Geometry: final body of the model. Coordinates: model frame, mm. Face numbers are marked on the shaded views. Give positions to 0.01 mm unless a question says otherwise; leave off trailing zeros. Loops run counter-clockwise (first coordinate to the right, second up) from the corner with the lowest first, then second, coordinate; pieces in that order, holes last. Notation, with made-up numbers: M 6,56 L 11,56 A22 cw 11,67 Z; hole C 56.5,-11.75 d8. An arc over 180 degrees is marked long. Put each result on its own line as item: value.
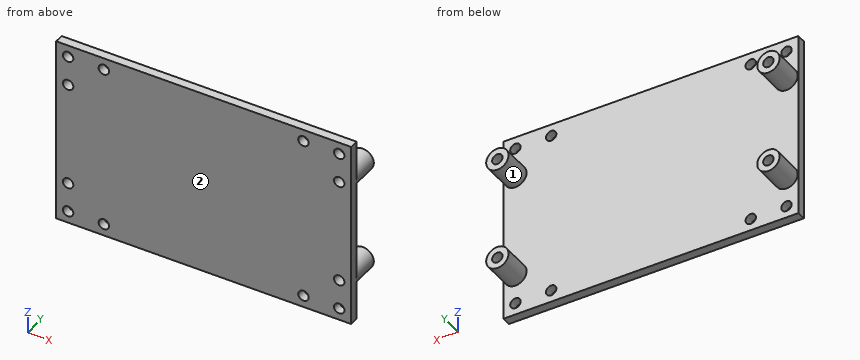
```python
from build123d import *

# Parameters (mm, degrees)
SKETCH1_W           = 99
SKETCH1_H           = 63
SKETCH1_R           = 3.75
SKETCH1_R_2         = 1.75
BOSS_EXTRUDE1_DEPTH = 3
SKETCH1_3_R         = 3.75
SKETCH1_3_R_2       = 1.75
BOSS_EXTRUDE2_DEPTH = 13


with BuildPart() as part:
    # Sketch1 → Boss-Extrude1 (new body)
    with BuildSketch(Plane(origin=(0, 0, 0), x_dir=(1, 0, 0), z_dir=(0, 1, 0))):
        Rectangle(SKETCH1_W, SKETCH1_H)
        with Locations(Location((-45.5, -17.5, 0), (0, 0, 270))):
            Circle(SKETCH1_R, mode=Mode.SUBTRACT)
        with Locations(Location((45.5, -17.5, 0), (0, 0, 270))):
            Circle(SKETCH1_R, mode=Mode.SUBTRACT)
        with Locations(Location((-45.5, 17.5, 0), (0, 0, 270))):
            Circle(SKETCH1_R, mode=Mode.SUBTRACT)
        with Locations(Location((45.5, 17.5, 0), (0, 0, 270))):
            Circle(SKETCH1_R, mode=Mode.SUBTRACT)
        with Locations(Location((45.5, 27.5, 0), (0, 0, 270))):
            Circle(SKETCH1_R_2, mode=Mode.SUBTRACT)
        with Locations(Location((-45.5, 27.5, 0), (0, 0, 270))):
            Circle(SKETCH1_R_2, mode=Mode.SUBTRACT)
        with Locations(Location((-33.5, 27.5, 0), (0, 0, 270))):
            Circle(SKETCH1_R_2, mode=Mode.SUBTRACT)
        with Locations(Location((33.5, 27.5, 0), (0, 0, 270))):
            Circle(SKETCH1_R_2, mode=Mode.SUBTRACT)
        with Locations(Location((45.5, -27.5, 0), (0, 0, 270))):
            Circle(SKETCH1_R_2, mode=Mode.SUBTRACT)
        with Locations(Location((-45.5, -27.5, 0), (0, 0, 270))):
            Circle(SKETCH1_R_2, mode=Mode.SUBTRACT)
        with Locations(Location((-33.5, -27.5, 0), (0, 0, 270))):
            Circle(SKETCH1_R_2, mode=Mode.SUBTRACT)
        with Locations(Location((33.5, -27.5, 0), (0, 0, 270))):
            Circle(SKETCH1_R_2, mode=Mode.SUBTRACT)
    extrude(amount=BOSS_EXTRUDE1_DEPTH)

    # Sketch1_3 → Boss-Extrude2 (add)
    # profile 1 of 4: a face of its own
    with BuildSketch(Plane(origin=(0, 0, 0), x_dir=(1, 0, 0), z_dir=(0, 1, 0))):
        with Locations(Location((-45.5, 17.5, 0), (0, 0, 90))):
            Circle(SKETCH1_3_R)
        with Locations(Location((-45.5, 17.5, 0), (0, 0, 90))):
            Circle(SKETCH1_3_R_2, mode=Mode.SUBTRACT)
    # profile 2 of 4: a face of its own
    with BuildSketch(Plane(origin=(0, 0, 0), x_dir=(1, 0, 0), z_dir=(0, 1, 0))):
        with Locations(Location((-45.5, -17.5, 0), (0, 0, 90))):
            Circle(SKETCH1_3_R)
        with Locations(Location((-45.5, -17.5, 0), (0, 0, 90))):
            Circle(SKETCH1_3_R_2, mode=Mode.SUBTRACT)
    # profile 3 of 4: a face of its own
    with BuildSketch(Plane(origin=(0, 0, 0), x_dir=(1, 0, 0), z_dir=(0, 1, 0))):
        with Locations(Location((45.5, -17.5, 0), (0, 0, 90))):
            Circle(SKETCH1_3_R)
        with Locations(Location((45.5, -17.5, 0), (0, 0, 90))):
            Circle(SKETCH1_3_R_2, mode=Mode.SUBTRACT)
    # profile 4 of 4: a face of its own
    with BuildSketch(Plane(origin=(0, 0, 0), x_dir=(1, 0, 0), z_dir=(0, 1, 0))):
        with Locations(Location((45.5, 17.5, 0), (0, 0, 90))):
            Circle(SKETCH1_3_R)
        with Locations(Location((45.5, 17.5, 0), (0, 0, 90))):
            Circle(SKETCH1_3_R_2, mode=Mode.SUBTRACT)
    extrude(amount=BOSS_EXTRUDE2_DEPTH)


solid = part.part
```
Item 1: Pin query (flat end, axial travel): pin 1 Ø1 at (x, z) = (21, -7.5) entering from +Y; pin 2 Ø3 at (y, z) = (7.5, 14.5) entering from -X. Return the tip coordinate at first contact, or that it passes through.
Output values:
pin 1: y = 3
pin 2: x = -48.94
Item 2: Section D-D on z = 17.5. Output: boundary loops of the cut face in (x, y).
Output values:
outline: M -49.5,0 L -47.25,0 L -47.25,13 L -49.25,13 L -49.25,3 L -49.5,3 Z; M -43.75,0 L 43.75,0 L 43.75,13 L 41.75,13 L 41.75,3 L -41.75,3 L -41.75,13 L -43.75,13 Z; M 47.25,0 L 49.5,0 L 49.5,3 L 49.25,3 L 49.25,13 L 47.25,13 Z
Item 3: Mould query, pull axis Z, two halves, no side actions, for the marked faces 1 and 2. Classes: pulls with the +Z half, pulls with the -Z half, needs draft (parallel to the pull), parting line crosses it, or undercut.
Output values:
face 1: undercut
face 2: needs draft
Item 4: Line query: probe 1 along Z at (x, y) = (-45.5, 3.75); probe 2 along X at (y, z) = (0.7, 27.5); probe 3 along X at (y, z) = (10.25, 17.5). Output: solid intervals per line, ascending. Write a range as [from, to].
Output values:
probe 1: [-21.25, -19.25], [-15.75, -13.75], [13.75, 15.75], [19.25, 21.25]
probe 2: [-49.5, -47.25], [-43.75, -35.25], [-31.75, 31.75], [35.25, 43.75], [47.25, 49.5]
probe 3: [-49.25, -47.25], [-43.75, -41.75], [41.75, 43.75], [47.25, 49.25]
Item 5: Section B-B on z = 27.5. Output: boundary loops of the cut face in (x, y), then the cut area to 3 significant figures.
Output values:
outline: M -49.5,0 L -47.25,0 L -47.25,3 L -49.5,3 Z; M -43.75,0 L -35.25,0 L -35.25,3 L -43.75,3 Z; M -31.75,0 L 31.75,0 L 31.75,3 L -31.75,3 Z; M 35.25,0 L 43.75,0 L 43.75,3 L 35.25,3 Z; M 47.25,0 L 49.5,0 L 49.5,3 L 47.25,3 Z
area: 255 mm²
Item 6: Section A-A on x = -45.5. Output: boundary loops of the cut face in (y, z).
Output values:
outline: M 0,-31.5 L 3,-31.5 L 3,-29.25 L 0,-29.25 Z; M 0,-25.75 L 3,-25.75 L 3,-21.25 L 13,-21.25 L 13,-19.25 L 0,-19.25 Z; M 0,-15.75 L 13,-15.75 L 13,-13.75 L 3,-13.75 L 3,13.75 L 13,13.75 L 13,15.75 L 0,15.75 Z; M 0,19.25 L 13,19.25 L 13,21.25 L 3,21.25 L 3,25.75 L 0,25.75 Z; M 0,29.25 L 3,29.25 L 3,31.5 L 0,31.5 Z
Item 7: Section C-C on y = 8.25. Output: boundary loops of the cut face in (x, z).
Output values:
outline: C -45.5,-17.5 d7.5; C -45.5,17.5 d7.5; C 45.5,-17.5 d7.5; C 45.5,17.5 d7.5; hole C -45.5,-17.5 d3.5; hole C -45.5,17.5 d3.5; hole C 45.5,-17.5 d3.5; hole C 45.5,17.5 d3.5
